Geometry check sheet. Reference: the model listing, model coordinates, mm. A direction names the side the tool comes from. Coordinates: 2 decimals unless noted, no trailing zeros. Write each loop counter-clockwise with the first axis right and the second up, starting at its lowest first coordinate (ties: lowest second). Pieces come first, ordered by that corner, then holes. Notation, with made-up numbers: (-16, 81) -> (23, 81) arc R22 cw to (23, 103) -> close; hole circle Ø10 at (88.25, 88). An arc over 180 degrees is marked (long way). Answer in a Markdown table with one row per item. Add a question column.
1. Scan lines: L1, parallel to Y at x = 1.5, z = 0.9; L2, parallel to X at y = 5, z = 1.25; L3, parallel to X at y = 1.75, z = 0.8. Record each from-to range of solid material in increasing order. Write a range as from..to.
2. Set-up check for faces 1 (the flat face through (-5.5, -4.1, 0.5)), 2 (the flat face through (-3.396, 8.335, 1.479)): record each of +Z, -Z, +X, -X, +Y, -Y from which the full face is reachable in a straight line by a thin tool's end or side.
3. Cross-section at A-A on z = 2.75. Record the cut outline in (x, y).
4. Depth check by flat-ended pin: P1, Ø1.9, axis at x = 5.5, y = -3.5, coming from the -Z side; P2, Ø0.6, axis at y = -3.5, z = 0, coming from the +X side; P3, Ø0.6, axis at x = 5, z = 0.5, coming from the +Y side; P4, Ø1.9, axis at x = 4.5, y = 4, coming from the -Z side. Enter the tip coordinate at first touch or a pass-through.
5. Cross-section at C-C on x = 5. Record the cut outline in (y, z).
6. Mould release check, pull along X, two halves, no side actions. Record for faces 3 (the flat face through (8.295, -3.492, 1.479)), 4 (the flat face through (5.5, -4.1, 0.5)), 5 (the flat face through (4.2, 5.2, 3)), 6 (the flat face through (-8.335, -3.396, 1.479)): pulls with the +X half, pulls with the -X half, needs draft (parallel to the pull), parting line crosses it, or undercut.
7. Cross-section at D-D on y = 4. Record the cut outline in (x, z), and give its area (3 significant figures).
8. Cross-section at B-B on y = 1. Record the cut outline in (x, z).
```python
from build123d import *

# Parameters (mm, degrees)
BOSS_EXTRUDE1_DEPTH     = 3
SKETCH4_W               = 12.3
SKETCH4_H               = 10.3
CUT_EXTRUDE2_DEPTH      = 0.5
FILLET1_R               = 0.5
F_1_2_20_TAPPED_HOLE1_D = 12.7
CUT_EXTRUDE3_REACH      = 5


with BuildPart() as part:
    # Sketch2 → Boss-Extrude1 (new body)
    with BuildSketch(Plane.XY):
        Polygon((0, 9.741529803), (-6.888301783, 6.888301783), (-9.741529803, 0), (-6.888301783, -6.888301783), (0, -9.741529803), (6.888301783, -6.888301783), (9.741529803, 0), (6.888301783, 6.888301783), align=None)
    extrude(amount=BOSS_EXTRUDE1_DEPTH)

    # Sketch4 → Cut-Extrude2 (cut)
    with BuildSketch(Plane(origin=(0, 0, 0), x_dir=(-1, 0, 0), z_dir=(0, 0, -1))):
        Rectangle(SKETCH4_W, SKETCH4_H)
    extrude(amount=-CUT_EXTRUDE2_DEPTH, mode=Mode.SUBTRACT)

    # Fillet1
    fillet1_edges = [part.edges().sort_by_distance(p)[0] for p in [
        (-6.15, 5.15, 0.25),
        (-6.15, -5.15, 0.25),
        (6.15, -5.15, 0.25),
        (6.15, 5.15, 0.25),
    ]]
    fillet(fillet1_edges, radius=FILLET1_R)

    # 1/2-20 Tapped Hole1 (through all)
    with Locations(Plane.XY.offset(3)):
        with Locations((0, 0)):
            Hole(F_1_2_20_TAPPED_HOLE1_D / 2)

    # Sketch7 → Cut-Extrude3 (cut, up to next)
    with BuildSketch(Plane(origin=(0, 0, 0), x_dir=(-1, 0, 0), z_dir=(0, 0, -1)), mode=Mode.PRIVATE) as cut_extrude3_sk1:
        Polygon((-6.888301783, -6.888301783), (6.888301783, -6.888301783), (0, -9.741529803), align=None)
    cut_extrude3_tool1 = extrude(cut_extrude3_sk1.sketch, amount=-CUT_EXTRUDE3_REACH, mode=Mode.PRIVATE) & part.part
    add(cut_extrude3_tool1.solids().sort_by_distance((0, -7.839378, 0))[0], mode=Mode.SUBTRACT)


solid = part.part
```
Results found:
| question | item | result |
|---|---|---|
| 1 | L1 | y = -6.89..-6.17, 6.17..9.12 |
| 1 | L2 | x = -7.67..-3.91, 3.91..7.67 |
| 1 | L3 | x = -9.02..-6.1, 6.1..9.02 |
| 2 | face 1 | -Z |
| 2 | face 2 | +Z, -Z, -X, +Y |
| 3 | outline | (-9.74, 0) -> (-6.89, -6.89) -> (6.89, -6.89) -> (9.74, 0) -> (6.89, 6.89) -> (0, 9.74) -> (-6.89, 6.89) -> close; hole circle Ø12.7 at (0, 0) |
| 4 | P1 | stops at z = 0 |
| 4 | P2 | stops at x = 8.42 |
| 4 | P3 | stops at y = 7.79 |
| 4 | P4 | stops at z = 0.5 |
| 5 | outline | (-6.89, 0) -> (-5.15, 0) -> (-5.15, 0.5) -> (-3.91, 0.5) -> (-3.91, 3) -> (-6.89, 3) -> close; (3.91, 0.5) -> (5.15, 0.5) -> (5.15, 0) -> (7.67, 0) -> (7.67, 3) -> (3.91, 3) -> close |
| 6 | face 3 | pulls with the +X half |
| 6 | face 4 | undercut |
| 6 | face 5 | needs draft |
| 6 | face 6 | pulls with the -X half |
| 7 | outline | (-8.08, 0) -> (-6.15, 0) -> (-6.15, 0.5) -> (-4.93, 0.5) -> (-4.93, 3) -> (-8.08, 3) -> close; (4.93, 0.5) -> (6.15, 0.5) -> (6.15, 0) -> (8.08, 0) -> (8.08, 3) -> (4.93, 3) -> close |
| 7 | area | 17.7 mm^2 |
| 8 | outline | (-9.33, 0) -> (-6.27, 0) -> (-6.27, 3) -> (-9.33, 3) -> close; (6.27, 0) -> (9.33, 0) -> (9.33, 3) -> (6.27, 3) -> close |
